```python
from build123d import *

# Parameters (mm, degrees)
CYLINDER001_R           = 1.5
CYLINDER001_DEPTH       = 5
CYLINDER001_PITCH_ANGLE = 90
CYLINDER002_R           = 1.5
CYLINDER002_DEPTH       = 5
CYLINDER002_PITCH_ANGLE = 90
CYLINDER003_R           = 1.5
CYLINDER003_DEPTH       = 5
CYLINDER003_PITCH_ANGLE = 90
CYLINDER004_R           = 1.5
CYLINDER004_DEPTH       = 5
CYLINDER004_ROLL_ANGLE  = 90.0000000001
CYLINDER005_R           = 1.5
CYLINDER005_DEPTH       = 5
CYLINDER005_ROLL_ANGLE  = 90.0000000001
CYLINDER006_R           = 1.5
CYLINDER006_DEPTH       = 5
CYLINDER006_ROLL_ANGLE  = 90.0000000001
CYLINDER007_R           = 1.5
CYLINDER007_DEPTH       = 5
CYLINDER007_ROLL_ANGLE  = 90.0000000001
CYLINDER_R              = 1.5
CYLINDER_DEPTH          = 5
CYLINDER_PITCH_ANGLE    = 90
BOX008_W                = 5.5
BOX008_H                = 2.5
BOX008_DEPTH            = 5.5
BOX008_PLACEMENT_ANGLE  = -90.0000000001
BOX009_W                = 5.5
BOX009_H                = 2.5
BOX009_DEPTH            = 5.5
BOX009_PLACEMENT_ANGLE  = -90.0000000001
BOX007_W                = 5.5
BOX007_H                = 2.5
BOX007_DEPTH            = 5.5
BOX007_PLACEMENT_ANGLE  = -90.0000000001
BOX006_W                = 5.5
BOX006_H                = 2.5
BOX006_DEPTH            = 5.5
BOX006_PLACEMENT_ANGLE  = -90.0000000001
BOX005_W                = 5.5
BOX005_H                = 2.5
BOX005_DEPTH            = 5.5
BOX004_W                = 5.5
BOX004_H                = 2.5
BOX004_DEPTH            = 5.5
BOX003_W                = 5.5
BOX003_H                = 2.5
BOX003_DEPTH            = 5.5
BOX002_W                = 5.5
BOX002_H                = 2.5
BOX002_DEPTH            = 5.5
BOX001_W                = 66.1999969482
BOX001_H                = 66.1999969482
BOX001_DEPTH            = 10
BOX_W                   = 76.1999969482
BOX_H                   = 76.1999969482
BOX_DEPTH               = 10


with BuildPart() as cylinder001:
    # Cylinder001 → Cylinder001 (new body)
    with BuildSketch(Plane.XY):
        Circle(CYLINDER001_R)
    extrude(amount=CYLINDER001_DEPTH)


with BuildPart() as cylinder001_1:
    # Cylinder001 pitch: moved
    add(cylinder001.part.rotate(Axis((0, 0, 0), (0, 1, 0)), CYLINDER001_PITCH_ANGLE))


with BuildPart() as cylinder001_2:
    # Cylinder001 placement: moved
    add(cylinder001_1.part.moved(Location((0, 50.8, 5))))


with BuildPart() as cylinder002:
    # Cylinder002 → Cylinder002 (new body)
    with BuildSketch(Plane.XY):
        Circle(CYLINDER002_R)
    extrude(amount=CYLINDER002_DEPTH)


with BuildPart() as cylinder002_1:
    # Cylinder002 pitch: moved
    add(cylinder002.part.rotate(Axis((0, 0, 0), (0, 1, 0)), CYLINDER002_PITCH_ANGLE))


with BuildPart() as cylinder002_2:
    # Cylinder002 placement: moved
    add(cylinder002_1.part.moved(Location((71.2, 50.8, 5))))


with BuildPart() as cylinder003:
    # Cylinder003 → Cylinder003 (new body)
    with BuildSketch(Plane.XY):
        Circle(CYLINDER003_R)
    extrude(amount=CYLINDER003_DEPTH)


with BuildPart() as cylinder003_1:
    # Cylinder003 pitch: moved
    add(cylinder003.part.rotate(Axis((0, 0, 0), (0, 1, 0)), CYLINDER003_PITCH_ANGLE))


with BuildPart() as cylinder003_2:
    # Cylinder003 placement: moved
    add(cylinder003_1.part.moved(Location((71.2, 25.4, 5))))


with BuildPart() as cylinder004:
    # Cylinder004 → Cylinder004 (new body)
    with BuildSketch(Plane.XY):
        Circle(CYLINDER004_R)
    extrude(amount=CYLINDER004_DEPTH)


with BuildPart() as cylinder004_1:
    # Cylinder004 roll: moved
    add(cylinder004.part.rotate(Axis((0, 0, 0), (1, 0, 0)), CYLINDER004_ROLL_ANGLE))


with BuildPart() as cylinder004_2:
    # Cylinder004 placement: moved
    add(cylinder004_1.part.moved(Location((25.4, 5, 5))))


with BuildPart() as cylinder005:
    # Cylinder005 → Cylinder005 (new body)
    with BuildSketch(Plane.XY):
        Circle(CYLINDER005_R)
    extrude(amount=CYLINDER005_DEPTH)


with BuildPart() as cylinder005_1:
    # Cylinder005 roll: moved
    add(cylinder005.part.rotate(Axis((0, 0, 0), (1, 0, 0)), CYLINDER005_ROLL_ANGLE))


with BuildPart() as cylinder005_2:
    # Cylinder005 placement: moved
    add(cylinder005_1.part.moved(Location((50.8, 5, 5))))


with BuildPart() as cylinder006:
    # Cylinder006 → Cylinder006 (new body)
    with BuildSketch(Plane.XY):
        Circle(CYLINDER006_R)
    extrude(amount=CYLINDER006_DEPTH)


with BuildPart() as cylinder006_1:
    # Cylinder006 roll: moved
    add(cylinder006.part.rotate(Axis((0, 0, 0), (1, 0, 0)), CYLINDER006_ROLL_ANGLE))


with BuildPart() as cylinder006_2:
    # Cylinder006 placement: moved
    add(cylinder006_1.part.moved(Location((50.8, 76.2, 5))))


with BuildPart() as cylinder007:
    # Cylinder007 → Cylinder007 (new body)
    with BuildSketch(Plane.XY):
        Circle(CYLINDER007_R)
    extrude(amount=CYLINDER007_DEPTH)


with BuildPart() as cylinder007_1:
    # Cylinder007 roll: moved
    add(cylinder007.part.rotate(Axis((0, 0, 0), (1, 0, 0)), CYLINDER007_ROLL_ANGLE))


with BuildPart() as cylinder007_2:
    # Cylinder007 placement: moved
    add(cylinder007_1.part.moved(Location((25.4, 76.2, 5))))


with BuildPart() as cylinder:
    # Cylinder → Cylinder (new body)
    with BuildSketch(Plane.XY):
        Circle(CYLINDER_R)
    extrude(amount=CYLINDER_DEPTH)


with BuildPart() as cylinder_1:
    # Cylinder pitch: moved
    add(cylinder.part.rotate(Axis((0, 0, 0), (0, 1, 0)), CYLINDER_PITCH_ANGLE))


with BuildPart() as cylinder_2:
    # Cylinder placement: moved
    add(cylinder_1.part.moved(Location((0, 25.4, 5))))


with BuildPart() as box008:
    # Box008 → Box008 (new body)
    with BuildSketch(Plane.XY):
        with Locations((2.75, 1.25)):
            Rectangle(BOX008_W, BOX008_H)
    extrude(amount=BOX008_DEPTH)


with BuildPart() as box008_1:
    # Box008 placement: moved
    add(box008.part.moved(Location((71.19, 28.15, 2.5))).rotate(Axis((71.19, 28.15, 2.5), (0, 0, 1)), BOX008_PLACEMENT_ANGLE))


with BuildPart() as box009:
    # Box009 → Box009 (new body)
    with BuildSketch(Plane.XY):
        with Locations((2.75, 1.25)):
            Rectangle(BOX009_W, BOX009_H)
    extrude(amount=BOX009_DEPTH)


with BuildPart() as box009_1:
    # Box009 placement: moved
    add(box009.part.moved(Location((71.19, 53.55, 2.5))).rotate(Axis((71.19, 53.55, 2.5), (0, 0, 1)), BOX009_PLACEMENT_ANGLE))


with BuildPart() as box007:
    # Box007 → Box007 (new body)
    with BuildSketch(Plane.XY):
        with Locations((2.75, 1.25)):
            Rectangle(BOX007_W, BOX007_H)
    extrude(amount=BOX007_DEPTH)


with BuildPart() as box007_1:
    # Box007 placement: moved
    add(box007.part.moved(Location((2.5, 53.55, 2.5))).rotate(Axis((2.5, 53.55, 2.5), (0, 0, 1)), BOX007_PLACEMENT_ANGLE))


with BuildPart() as box006:
    # Box006 → Box006 (new body)
    with BuildSketch(Plane.XY):
        with Locations((2.75, 1.25)):
            Rectangle(BOX006_W, BOX006_H)
    extrude(amount=BOX006_DEPTH)


with BuildPart() as box006_1:
    # Box006 placement: moved
    add(box006.part.moved(Location((2.5, 28.15, 2.5))).rotate(Axis((2.5, 28.15, 2.5), (0, 0, 1)), BOX006_PLACEMENT_ANGLE))


with BuildPart() as box005:
    # Box005 → Box005 (new body)
    with BuildSketch(Plane(origin=(22.65, 71.19, 2.25), x_dir=(1, 0, 0), z_dir=(0, 0, 1))):
        with Locations((2.75, 1.25)):
            Rectangle(BOX005_W, BOX005_H)
    extrude(amount=BOX005_DEPTH)


with BuildPart() as box004:
    # Box004 → Box004 (new body)
    with BuildSketch(Plane(origin=(48.05, 71.19, 2.25), x_dir=(1, 0, 0), z_dir=(0, 0, 1))):
        with Locations((2.75, 1.25)):
            Rectangle(BOX004_W, BOX004_H)
    extrude(amount=BOX004_DEPTH)


with BuildPart() as box003:
    # Box003 → Box003 (new body)
    with BuildSketch(Plane(origin=(48.05, 2.5, 2.25), x_dir=(1, 0, 0), z_dir=(0, 0, 1))):
        with Locations((2.75, 1.25)):
            Rectangle(BOX003_W, BOX003_H)
    extrude(amount=BOX003_DEPTH)


with BuildPart() as box002:
    # Box002 → Box002 (new body)
    with BuildSketch(Plane(origin=(22.65, 2.5, 2.25), x_dir=(1, 0, 0), z_dir=(0, 0, 1))):
        with Locations((2.75, 1.25)):
            Rectangle(BOX002_W, BOX002_H)
    extrude(amount=BOX002_DEPTH)


with BuildPart() as box001:
    # Box001 → Box001 (new body)
    with BuildSketch(Plane(origin=(5, 5, 0), x_dir=(1, 0, 0), z_dir=(0, 0, 1))):
        with Locations((33.0999984741, 33.0999984741)):
            Rectangle(BOX001_W, BOX001_H)
    extrude(amount=BOX001_DEPTH)


with BuildPart() as cut016:
    # Box → Box (new body)
    with BuildSketch(Plane.XY):
        with Locations((38.0999984741, 38.0999984741)):
            Rectangle(BOX_W, BOX_H)
    extrude(amount=BOX_DEPTH)

    # Cut: cut Box001
    add(box001.part, mode=Mode.SUBTRACT)

    # Cut001: cut Box002
    add(box002.part, mode=Mode.SUBTRACT)

    # Cut002: cut Box003
    add(box003.part, mode=Mode.SUBTRACT)

    # Cut003: cut Box004
    add(box004.part, mode=Mode.SUBTRACT)

    # Cut004: cut Box005
    add(box005.part, mode=Mode.SUBTRACT)

    # Cut005: cut Box006
    add(box006_1.part, mode=Mode.SUBTRACT)

    # Cut006: cut Box007
    add(box007_1.part, mode=Mode.SUBTRACT)

    # Cut007: cut Box009
    add(box009_1.part, mode=Mode.SUBTRACT)

    # Cut008: cut Box008
    add(box008_1.part, mode=Mode.SUBTRACT)

    # Cut009: cut Cylinder
    add(cylinder_2.part, mode=Mode.SUBTRACT)

    # Cut010: cut Cylinder007
    add(cylinder007_2.part, mode=Mode.SUBTRACT)

    # Cut011: cut Cylinder006
    add(cylinder006_2.part, mode=Mode.SUBTRACT)

    # Cut012: cut Cylinder005
    add(cylinder005_2.part, mode=Mode.SUBTRACT)

    # Cut013: cut Cylinder004
    add(cylinder004_2.part, mode=Mode.SUBTRACT)

    # Cut014: cut Cylinder003
    add(cylinder003_2.part, mode=Mode.SUBTRACT)

    # Cut015: cut Cylinder002
    add(cylinder002_2.part, mode=Mode.SUBTRACT)

    # Cut016: cut Cylinder001
    add(cylinder001_2.part, mode=Mode.SUBTRACT)


solid = cut016.part
```
Here's how the part is built. I have some questions about the finished solid (model axes, mm). A direction names the side the tool comes from. Round coordinates to 2 decimals unless told otherwise and drop trailing zeros. Order: outer loops, then holes, each group sorted by start corner. A loop starts at its lowest first (then second) coordinate and runs counter-clockwise, first axis right, second up. Notation, with made-up numbers: M 75.25,72 L 117.25,72 A12 ccw 117.25,91 Z; hole C 10,34.25 d5. An arc over 180 degrees is marked long. One line per question, with ' | ' between items.
1) I want a section at A-A, the plane x = 37.5. Write out the boundary of the cut face in (y, z), then the cut area to 3 significant figures.
Working result:
outline: M 0,0 L 5,0 L 5,10 L 0,10 Z; M 71.2,0 L 76.2,0 L 76.2,10 L 71.2,10 Z | area: 100 mm²
2) If we mould it in two halves opening along Y, with no side actions, what happens to faces 4 (the face through (72, 25, 2.5)), 5 (the face through (52.23, 1.27, 5.45))? For each: +Y half, -Y half, draft (parallel to the pull), parting line (faces both ways), or undercut.
Working result:
face 4: undercut | face 5: draft
3) I need wall thicknesses on line 1 along X through (y, z) = (1.45, 5); line 2 along Y through (x, z) = (55, 7). Which ranges of each line are inside material? Lowest first, please.
Working result:
line 1: 0 to 23.9, 26.9 to 49.3, 52.3 to 76.2 | line 2: 0 to 5, 71.2 to 76.2
4) I want a section at D-D, the plane x = 25.4. Write out the boundary of the cut face in (y, z), then the cut area to 3 significant figures.
Working result:
outline: M 0,0 L 5,0 L 5,2.25 L 2.5,2.25 L 2.5,3.5 L 0,3.5 Z; M 0,6.5 L 2.5,6.5 L 2.5,7.75 L 5,7.75 L 5,10 L 0,10 Z; M 71.2,0 L 76.2,0 L 76.2,3.5 L 73.69,3.5 L 73.69,2.25 L 71.2,2.25 Z; M 71.2,7.75 L 73.69,7.75 L 73.69,6.5 L 76.2,6.5 L 76.2,10 L 71.2,10 Z | area: 57.5 mm²
5) For faces 1 (the face through (4, 51, 8)), 2 (the face through (74.927, 49.336, 5.325)), 3 (the face through (38, 5, 5)), which set-ups out of +Z, -Z, +X, -X, +Y, -Y let a thin tool reach every point of the face, with its end or its side?
Working result:
face 1: none | face 2: +X, -X | face 3: +Z, -Z
6) I want a section at C-C, the plane y = 50.8. Write out the boundary of the cut face in (x, z).
Working result:
outline: M 0,0 L 5,0 L 5,2.5 L 2.5,2.5 L 2.5,3.5 L 0,3.5 Z; M 0,6.5 L 2.5,6.5 L 2.5,8 L 5,8 L 5,10 L 0,10 Z; M 71.2,0 L 76.2,0 L 76.2,3.5 L 73.69,3.5 L 73.69,2.5 L 71.2,2.5 Z; M 71.2,8 L 73.69,8 L 73.69,6.5 L 76.2,6.5 L 76.2,10 L 71.2,10 Z
